Source: CAD feature listing. Evaluate the final solid. Frame: model axes, mm. A direction names the side the tool comes from. Coordinates: 2 decimals unless noted, no trailing zeros. Order: outer loops, then holes, each group sorted by start corner. A loop starts at its lowest first (then second) coordinate and runs counter-clockwise, first axis right, second up.
```python
from build123d import *

# Parameters (mm, degrees)
CYLINDER541_R               = 1.5
CYLINDER541_DEPTH           = 20
CYLINDER541_PLACEMENT_ANGLE = -112.5
CYLINDER542_R               = 1.5
CYLINDER542_DEPTH           = 20
CYLINDER542_PLACEMENT_ANGLE = 112.5
CYLINDER543_R               = 1.5
CYLINDER543_DEPTH           = 20
CYLINDER543_PLACEMENT_ANGLE = 112.5
CYLINDER540_R               = 1.5
CYLINDER540_DEPTH           = 20
CYLINDER540_PLACEMENT_ANGLE = -112.5
BOX742_W                    = 6
BOX742_H                    = 6
BOX742_DEPTH                = 2
BOX743_W                    = 6
BOX743_H                    = 6
BOX743_DEPTH                = 2
BOX744_W                    = 6
BOX744_H                    = 6
BOX744_DEPTH                = 2
BOX741_W                    = 6
BOX741_H                    = 6
BOX741_DEPTH                = 2
CYLINDER538_R               = 3
CYLINDER538_DEPTH           = 3
CYLINDER537_R               = 3
CYLINDER537_DEPTH           = 3
CYLINDER536_R               = 3
CYLINDER536_DEPTH           = 3
CYLINDER539_R               = 3
CYLINDER539_DEPTH           = 3
CYLINDER535_R               = 1.6
CYLINDER535_DEPTH           = 80
CYLINDER533_R               = 1.6
CYLINDER533_DEPTH           = 80
CYLINDER534_R               = 1.6
CYLINDER534_DEPTH           = 80
CYLINDER532_R               = 1.6
CYLINDER532_DEPTH           = 80
CYLINDER531_R               = 6
CYLINDER531_DEPTH           = 20
CYLINDER530_R               = 11
CYLINDER530_DEPTH           = 7
CYLINDER529_R               = 8
CYLINDER529_DEPTH           = 20
BOX740_W                    = 16
BOX740_H                    = 19
BOX740_DEPTH                = 50
BOX739_W                    = 26
BOX739_H                    = 34
BOX739_DEPTH                = 36
CUT681_PLACEMENT_ANGLE      = 180


with BuildPart() as obj1:
    # Cylinder541 → Cylinder541 (new body)
    with BuildSketch(Plane.XY):
        Circle(CYLINDER541_R)
    extrude(amount=CYLINDER541_DEPTH)


with BuildPart() as obj1_1:
    # Cylinder541 placement: moved
    add(obj1.part.moved(Location((-8, 34, 51))).rotate(Axis((-8, 34, 51), (0, 0, 1)), CYLINDER541_PLACEMENT_ANGLE))


with BuildPart() as obj2:
    # Cylinder542 → Cylinder542 (new body)
    with BuildSketch(Plane.XY):
        Circle(CYLINDER542_R)
    extrude(amount=CYLINDER542_DEPTH)


with BuildPart() as obj2_1:
    # Cylinder542 placement: moved
    add(obj2.part.moved(Location((8, 62, 51))).rotate(Axis((8, 62, 51), (0, 0, -1)), CYLINDER542_PLACEMENT_ANGLE))


with BuildPart() as obj3:
    # Cylinder543 → Cylinder543 (new body)
    with BuildSketch(Plane.XY):
        Circle(CYLINDER543_R)
    extrude(amount=CYLINDER543_DEPTH)


with BuildPart() as obj3_1:
    # Cylinder543 placement: moved
    add(obj3.part.moved(Location((-8, 62, 51))).rotate(Axis((-8, 62, 51), (0, 0, -1)), CYLINDER543_PLACEMENT_ANGLE))


with BuildPart() as compound423:
    # Cylinder540 → Cylinder540 (new body)
    with BuildSketch(Plane.XY):
        Circle(CYLINDER540_R)
    extrude(amount=CYLINDER540_DEPTH)


with BuildPart() as compound423_1:
    # Cylinder540 placement: moved
    add(compound423.part.moved(Location((8, 34, 51))).rotate(Axis((8, 34, 51), (0, 0, 1)), CYLINDER540_PLACEMENT_ANGLE))

    # Compound423: union obj1, obj2, obj3
    add(obj1_1.part)
    add(obj2_1.part)
    add(obj3_1.part)


with BuildPart() as compound423_2:
    # Compound423 placement: moved
    add(compound423_1.part.moved(Location((0, 0, 5))))


with BuildPart() as krychle741:
    # Box742 → Box742 (new body)
    with BuildSketch(Plane(origin=(5, 59, 53), x_dir=(1, 0, 0), z_dir=(0, 0, 1))):
        with Locations((3, 3)):
            Rectangle(BOX742_W, BOX742_H)
    extrude(amount=BOX742_DEPTH)


with BuildPart() as krychle742:
    # Box743 → Box743 (new body)
    with BuildSketch(Plane(origin=(5, 31, 53), x_dir=(1, 0, 0), z_dir=(0, 0, 1))):
        with Locations((3, 3)):
            Rectangle(BOX743_W, BOX743_H)
    extrude(amount=BOX743_DEPTH)


with BuildPart() as krychle743:
    # Box744 → Box744 (new body)
    with BuildSketch(Plane(origin=(-11, 31, 53), x_dir=(1, 0, 0), z_dir=(0, 0, 1))):
        with Locations((3, 3)):
            Rectangle(BOX744_W, BOX744_H)
    extrude(amount=BOX744_DEPTH)


with BuildPart() as compound422:
    # Box741 → Box741 (new body)
    with BuildSketch(Plane(origin=(-11, 59, 53), x_dir=(1, 0, 0), z_dir=(0, 0, 1))):
        with Locations((3, 3)):
            Rectangle(BOX741_W, BOX741_H)
    extrude(amount=BOX741_DEPTH)

    # Compound422: union Krychle741, Krychle742, Krychle743
    add(krychle741.part)
    add(krychle742.part)
    add(krychle743.part)


with BuildPart() as compound422_1:
    # Compound422 placement: moved
    add(compound422.part.moved(Location((0, 0, 4))))


with BuildPart() as obj4:
    # Cylinder538 → Cylinder538 (new body)
    with BuildSketch(Plane(origin=(-10, 80, 31), x_dir=(1, 0, 0), z_dir=(0, -1, 0))):
        Circle(CYLINDER538_R)
    extrude(amount=CYLINDER538_DEPTH)


with BuildPart() as obj5:
    # Cylinder537 → Cylinder537 (new body)
    with BuildSketch(Plane(origin=(10, 80, 55), x_dir=(1, 0, 0), z_dir=(0, -1, 0))):
        Circle(CYLINDER537_R)
    extrude(amount=CYLINDER537_DEPTH)


with BuildPart() as obj6:
    # Cylinder536 → Cylinder536 (new body)
    with BuildSketch(Plane(origin=(10, 80, 31), x_dir=(1, 0, 0), z_dir=(0, -1, 0))):
        Circle(CYLINDER536_R)
    extrude(amount=CYLINDER536_DEPTH)


with BuildPart() as compound421:
    # Cylinder539 → Cylinder539 (new body)
    with BuildSketch(Plane(origin=(-10, 80, 55), x_dir=(1, 0, 0), z_dir=(0, -1, 0))):
        Circle(CYLINDER539_R)
    extrude(amount=CYLINDER539_DEPTH)

    # Compound421: union obj4, obj5, obj6
    add(obj4.part)
    add(obj5.part)
    add(obj6.part)


with BuildPart() as compound421_1:
    # Compound421 placement: moved
    add(compound421.part.moved(Location((0, -8, 0))))


with BuildPart() as obj7:
    # Cylinder535 → Cylinder535 (new body)
    with BuildSketch(Plane(origin=(-10, 80, 31), x_dir=(1, 0, 0), z_dir=(0, -1, 0))):
        Circle(CYLINDER535_R)
    extrude(amount=CYLINDER535_DEPTH)


with BuildPart() as obj8:
    # Cylinder533 → Cylinder533 (new body)
    with BuildSketch(Plane(origin=(10, 80, 55), x_dir=(1, 0, 0), z_dir=(0, -1, 0))):
        Circle(CYLINDER533_R)
    extrude(amount=CYLINDER533_DEPTH)


with BuildPart() as obj9:
    # Cylinder534 → Cylinder534 (new body)
    with BuildSketch(Plane(origin=(10, 80, 31), x_dir=(1, 0, 0), z_dir=(0, -1, 0))):
        Circle(CYLINDER534_R)
    extrude(amount=CYLINDER534_DEPTH)


with BuildPart() as compound420:
    # Cylinder532 → Cylinder532 (new body)
    with BuildSketch(Plane(origin=(-10, 80, 55), x_dir=(1, 0, 0), z_dir=(0, -1, 0))):
        Circle(CYLINDER532_R)
    extrude(amount=CYLINDER532_DEPTH)

    # Compound420: union obj7, obj8, obj9
    add(obj7.part)
    add(obj8.part)
    add(obj9.part)


with BuildPart() as obj10:
    # Cylinder531 → Cylinder531 (new body)
    with BuildSketch(Plane(origin=(0, 73, 43), x_dir=(1, 0, 0), z_dir=(0, -1, 0))):
        Circle(CYLINDER531_R)
    extrude(amount=CYLINDER531_DEPTH)


with BuildPart() as obj11:
    # Cylinder530 → Cylinder530 (new body)
    with BuildSketch(Plane(origin=(0, 65, 43), x_dir=(1, 0, 0), z_dir=(0, -1, 0))):
        Circle(CYLINDER530_R)
    extrude(amount=CYLINDER530_DEPTH)


with BuildPart() as obj12:
    # Cylinder529 → Cylinder529 (new body)
    with BuildSketch(Plane(origin=(0, 40, 43), x_dir=(1, 0, 0), z_dir=(0, -1, 0))):
        Circle(CYLINDER529_R)
    extrude(amount=CYLINDER529_DEPTH)


with BuildPart() as krychle739:
    # Box740 → Box740 (new body)
    with BuildSketch(Plane(origin=(-8, 37, 30), x_dir=(1, 0, 0), z_dir=(0, 0, 1))):
        with Locations((8, 9.5)):
            Rectangle(BOX740_W, BOX740_H)
    extrude(amount=BOX740_DEPTH)


with BuildPart() as t_mini_small_box:
    # Box739 → Box739 (new body)
    with BuildSketch(Plane(origin=(-13, 31, 25), x_dir=(1, 0, 0), z_dir=(0, 0, 1))):
        with Locations((13, 17)):
            Rectangle(BOX739_W, BOX739_H)
    extrude(amount=BOX739_DEPTH)

    # Cut675: cut Krychle739
    add(krychle739.part, mode=Mode.SUBTRACT)

    # Cut076: cut obj12
    add(obj12.part, mode=Mode.SUBTRACT)

    # Cut676: cut obj11
    add(obj11.part, mode=Mode.SUBTRACT)

    # Cut677: cut obj10
    add(obj10.part, mode=Mode.SUBTRACT)

    # Cut678: cut Compound420
    add(compound420.part, mode=Mode.SUBTRACT)

    # Cut679: cut Compound421
    add(compound421_1.part, mode=Mode.SUBTRACT)

    # Cut680: cut Compound422
    add(compound422_1.part, mode=Mode.SUBTRACT)

    # Cut681: cut Compound423
    add(compound423_2.part, mode=Mode.SUBTRACT)


with BuildPart() as t_mini_small_box_1:
    # Cut681 placement: moved
    add(t_mini_small_box.part.moved(Location((0, 2, -55))).rotate(Axis((0, 2, -55), (1, 0, 0)), CUT681_PLACEMENT_ANGLE))


solid = t_mini_small_box_1.part
```
1. Section query B-B on x = 0. Return loops of the section in (y, z).
Findings:
outline: (-63, -116) - (-54, -116) - (-54, -104) - (-56, -104) - (-56, -109) - (-63, -109) - close; (-63, -87) - (-56, -87) - (-56, -92) - (-54, -92) - (-54, -85) - (-35, -85) - (-35, -90) - (-29, -90) - (-29, -80) - (-63, -80) - close; (-35, -116) - (-29, -116) - (-29, -106) - (-35, -106) - close
2. Section query C-C on y = -51. Return loops of the section in (x, z), plus the area to 3 significant figures.
Findings:
outline: (-13, -116) - (-8, -116) - (-8, -85) - (8, -85) - (8, -116) - (13, -116) - (13, -80) - (-13, -80) - close; hole circle Ø3.2 at (-10, -110); hole circle Ø3.2 at (-10, -86); hole circle Ø3.2 at (10, -110); hole circle Ø3.2 at (10, -86)
area: 408 mm2
3. Access query for faces 5 (the face through (6.6, -33.4, -112)), 6 (the face through (0, -45, -85)), 7 (the face through (-11.18, -46.24, -87.08)), 8 (the face through (-8, -57, -113)). Directions: +Z, -Z, +X, -X, +Y, -Y. A direction counts if a zero-diameter tool reaches every point of the face in a straight line with its end or side. Return the directions, or none.
Findings:
face 5: +Y
face 6: -Z
face 7: +Y, -Y
face 8: -Y
4. Pin query (flat end, axial travel): P1, Ø3, axis at x = 1, y = -47.5, coming from the -Z side; P2, Ø1.6, axis at x = 10, z = -113, coming from the +Y side; P3, Ø11, axis at x = 0, z = -98, coming from the -Y side; P4, Ø0.7, axis at x = 7.5, y = -31.5, coming from the -Z side. Return the tip coordinate at first contact, or that it passes through.
Findings:
P1: stops at z = -85
P2: stops at y = -35
P3: passes through
P4: stops at z = -111
5. Section query A-A on z = -86. Return loops of the section in (x, y).
Findings:
outline: (-13, -63) - (-11.6, -63) - (-11.6, -29) - (-13, -29) - close; (-8.4, -63) - (8.4, -63) - (8.4, -29) - (-8.4, -29) - close; (11.6, -63) - (13, -63) - (13, -29) - (11.6, -29) - close; hole (-8, -54) - (8, -54) - (8, -35) - (-8, -35) - close
6. Draft query along Y for faces 1 (the face through (8, -57, -113)), 2 (the face through (-9.4, -61.4, -112)), 3 (the face through (-8, -32, -111)), 4 (the face through (8, -60, -111)). Return one class per face: released by +Y, released by -Y, zero draft, split by the parting line, or undercut.
Findings:
face 1: released by -Y
face 2: zero draft
face 3: undercut
face 4: undercut
7. Section query D-D on y = -59.5. Count the separate pieces of the cut face and the enclosed holes in it, plus the area to 3 significant figures.
Findings:
separate pieces: 1
enclosed holes: 3
area: 483 mm2
8. Ray query, line 1 (X direction, y = -32, z = -114.55); line 2 (Z direction, x = 10, y = -42); line 3 (X direction, y = -51.5, z = -86). Return the intervals inside material, ascending.
Findings:
line 1: x = -13 to -9.5, -6.5 to 6.5, 9.5 to 13
line 2: z = -116 to -111.6, -108.4 to -87.6, -84.4 to -80
line 3: x = -13 to -11.6, -8.4 to -8, 8 to 8.4, 11.6 to 13
